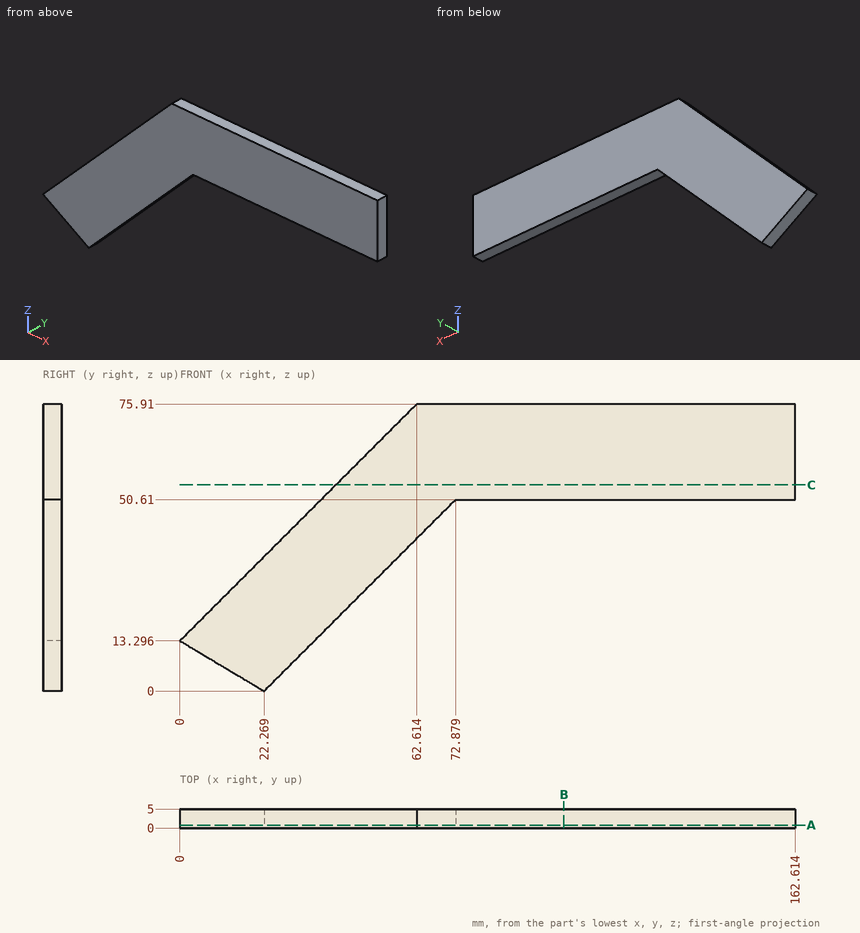
Drawing for the job (mm, zero at the part's lowest x, y, z). Round coordinates to 2 decimals unless told otherwise and drop trailing zeros. Loops run counter-clockwise (first coordinate to the right, second up) from the corner with the lowest first, then second, coordinate; pieces in that order, holes last. Notation, with made-up numbers: (-10, 24.25) - (48, 24.25) arc R21 cw to (48, 29.25) - close; hole circle Ø6 at (-30.75, 58.25). An arc over 180 degrees is marked (long way). Return JSON: item names as keys, results as strings. Group by question number.
Q1. Flat gauge pins, fed straight in: pin 1 Ø5 at (x, z) = (71.5, 52.5) entering from -Y; pin 2 Ø2 at (y, z) = (0.5, 57) entering from -X (1 decimal); pin 3 Ø3 at (x, y) = (53.5, 3) entering from -Z. Where does each tip first touch, or does it go through?
Q2. Band-saw the part on B-B on x = 101.5. Give the cut face in (y, z).
Q3. Drill centre lines: line 1 along Z through (x, y) = (136.5, 4.4); line 2 along X through (y, z) = (3.65, 10.5) (1 decimal); line 3 along X through (y, z) = (4.2, 52.5) (1 decimal). Where is each one in solid material? Low to high. Write a range as [from, to].
Q4. Band-saw the part on A-A on y = 0.8. Give the cut face in (x, z).
Q5. Band-saw the part on C-C on z = 54.5. Give the cut face in (x, y), plus the area to 3 significant figures.
Solutions:
{
 "1": {"pin 1": "stops at y = 0", "pin 2": "stops at x = 42.7", "pin 3": "stops at z = 29.73"},
 "2": {"outline": "(0, 50.61) - (5, 50.61) - (5, 75.91) - (0, 75.91) - close"},
 "3": {"line 1": "z = [50.61, 75.91]", "line 2": "x = [4.7, 32.8]", "line 3": "x = [39.2, 162.6]"},
 "4": {"outline": "(0, 13.3) - (22.27, 0) - (72.88, 50.61) - (162.61, 50.61) - (162.61, 75.91) - (62.61, 75.91) - close"},
 "5": {"outline": "(41.2, 0) - (162.61, 0) - (162.61, 5) - (41.2, 5) - close", "area": "607 mm^2"}
}
